Geometry: final body of the model. Coordinates: model frame, mm. Face numbers are marked on the shaded views. A direction names the side the tool comes from. Give positions to 0.01 mm unless a question says otherwise; leave off trailing zeros. Loops run counter-clockwise (first coordinate to the right, second up) from the corner with the lowest first, then second, coordinate; pieces in that order, holes last. Notation, with made-up numbers: (86.25, -12.75) -> (130.25, -12.75) arc R26 ccw to (130.25, 3.25) -> close; hole circle Ø4 at (34.25, 50). An arc over 180 degrees is marked (long way). One line per question, with ' | ' between items. Start each with the question number.
Item 1: Material intervals for line 1 along Y through (x, z) = (54.5, -25); line 2 along Z through (x, y) = (54, -4); line 3 along X through (y, z) = (-21, -17), sorted ascending. Write a range as [from, to].
Item 2: Section B-B on x = 30. Return loops of the section in (y, z).
Item 3: Section A-A on z = -22. Return loops of the section in (x, y).
Item 4: Section D-D on x = -24.5. Return loops of the section in (y, z), then the cut area to 3 significant figures.
Item 5: Set-up query: the marked faces 1, 2 and 3. Return all of +Z, -Z, +X, -X, +Y, -Y with unobstructed straight access to the full face (end or side cutting, diameter ignored); none if empty.
Item 6: Section C-C on y = -3. Return loops of the section in (x, z), then the cut area to 3 significant figures.
Item 7: Pin query (flat end, axial travel): P1, Ø9.5, axis at x = 17.5, y = -8, coming from the +Z side; P2, Ø3, axis at x = -36.5, y = -10.5, coming from the +Z side; P3, Ø12, axis at x = -27.5, y = -29, coming from the +Z side; P4, Ø1.5, axis at x = 38, z = 1.5, coming from the +Y side. Return the tip coordinate at first contact, or that it passes through.
from build123d import *

# Parameters (mm, degrees)
F1_DEPTH = 38.1
F2_DEPTH = 19.05


with BuildPart() as f1:
    # F0 (on Front) → F1 (new body)
    with BuildSketch(Plane.XZ):
        Polygon((-63.5, 31.75), (-63.5, -31.75), (63.5, -31.75), (0, 0), align=None)
    extrude(amount=F1_DEPTH)

    # F0 (on Front) → F2 (join)
    with BuildSketch(Plane.XZ):
        Polygon((-63.5, 31.75), (-63.5, -31.75), (63.5, -31.75), (0, 0), align=None)
        Polygon((0, 0), (63.5, -31.75), (63.5, 0), align=None)
    extrude(amount=F2_DEPTH)


solid = f1.part
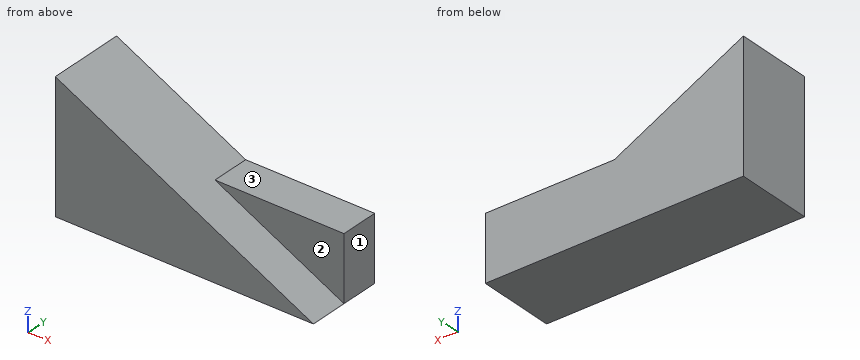
Result sheet:
1) line 1: y = [-19.05, 0] | line 2: z = [-31.75, 0] | line 3: x = [-63.5, 34]
2) outline: (-38.1, -31.75) -> (0, -31.75) -> (0, 0) -> (-19.05, 0) -> (-19.05, -15) -> (-38.1, -15) -> close
3) outline: (-63.5, -38.1) -> (44, -38.1) -> (44, -19.05) -> (63.5, -19.05) -> (63.5, 0) -> (-63.5, 0) -> close
4) outline: (-38.1, -31.75) -> (0, -31.75) -> (0, 12.25) -> (-38.1, 12.25) -> close | area: 1,680 mm²
5) face 1: +Z, -Z, +X, +Y, -Y | face 2: +Z, +X, -Y | face 3: +Z, +X, +Y, -Y
6) outline: (-63.5, -31.75) -> (63.5, -31.75) -> (63.5, 0) -> (0, 0) -> (-63.5, 31.75) -> close | area: 5,040 mm²
7) P1: stops at z = 0 | P2: stops at z = 19 | P3: stops at z = 16.75 | P4: passes through
